Geometry: final body of the model. Coordinates: model frame, mm. Face numbers are marked on the shaded views. Give positions to 0.01 mm unless a question says otherwise; leave off trailing zeros. Loops run counter-clockwise (first coordinate to the right, second up) from the corner with the lowest first, then second, coordinate; pieces in that order, holes last.
```python
from build123d import *

# Parameters (mm, degrees)
SKETCH1_R               = 12.7
BOSS_EXTRUDE1_DEPTH     = 19.05
SHELL1_T                = -3.175
SKETCH4_R               = 1.2446
CUT_EXTRUDE1_DEPTH      = 27.181720723
CUT_EXTRUDE1_DEPTH_BACK = 27.181720723
SKETCH7_R               = 10.8712
SKETCH7_R_2             = 9.525
CUT_EXTRUDE2_DEPTH      = 2.3622


with BuildPart() as part:
    # Sketch1 → Boss-Extrude1 (new body)
    with BuildSketch(Plane.XY):
        Circle(SKETCH1_R)
    extrude(amount=-BOSS_EXTRUDE1_DEPTH)

    # Shell1
    shell1_openings = [part.faces().sort_by_distance(p)[0] for p in [
        (0, 0, -19.05),
    ]]
    offset(amount=SHELL1_T, openings=shell1_openings, kind=Kind.INTERSECTION)

    # Sketch4 → Cut-Extrude1 (cut, two sides)
    with BuildSketch(Plane(origin=(0, 0, 0), x_dir=(0, 0, -1), z_dir=(1, 0, 0))) as cut_extrude1_sk:
        with Locations((13.0175, 0)):
            Circle(SKETCH4_R)
    extrude(amount=CUT_EXTRUDE1_DEPTH, mode=Mode.SUBTRACT)
    extrude(cut_extrude1_sk.sketch, amount=-CUT_EXTRUDE1_DEPTH_BACK, mode=Mode.SUBTRACT)

    # Sketch7 → Cut-Extrude2 (cut)
    with BuildSketch(Plane(origin=(0, 0, -17.78), x_dir=(-1, 0, 0), z_dir=(0, 0, -1))):
        Circle(SKETCH7_R)
        with Locations(Location((0, 0, 0), (0, 0, 180))):
            Circle(SKETCH7_R_2, mode=Mode.SUBTRACT)
    extrude(amount=-CUT_EXTRUDE2_DEPTH, mode=Mode.SUBTRACT)


solid = part.part
```
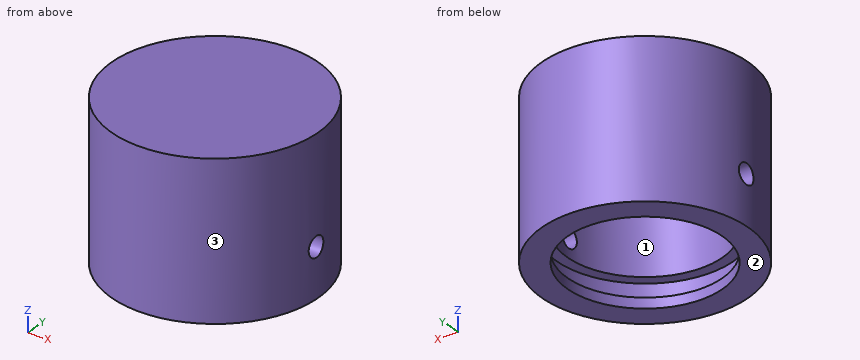
Q1. Mould query, pull axis Y, two halves, no side actions, for the marked faces 1, 2 and 3. Classes: +Y half, -Y half, draft (parallel to the pull), parting line (faces both ways), or undercut.
Q2. Section query C-C, the plane z = -16.25. Return loops of the section in (x, y), and give its area (3 significant figures).
Q3. Section query D-D, the plane z = -13. Return loops of the section in (x, y) (3 decimals), and give its area (3 significant figures).
Q4. Pin query (flat end, axial travel): pin 1 Ø3 at (x, y) = (-2, -5) entering from -Z (3 decimals); pin 2 Ø3 at (x, z) = (-7.5, -9.5) entering from +Y; pin 3 Ø4 at (x, z) = (4.5, -9) entering from +Y. Return the tip coordinate at first contact, or that it passes through.
Q5. Material intervals for probe 1 along Y at (x, z) = (0, -18.4) (3 decimals); probe 2 along Y at (x, z) = (0, -16.55), sorted ascending.
Q6. Section query B-B, the plane x = 0. Return loops of the section in (y, z) (3 decimals), and give its area (3 significant figures).
Q7. Section query A-A, the plane y = 0. Return loops of the section in (x, z) (3 decimals).
Resolved:
1. face 1: undercut
1. face 2: draft
1. face 3: parting line
2. outline: circle Ø25.4 at (0, 0); hole circle Ø21.74 at (0, 0)
2. area: 135 mm2
3. outline: (-12.639, -1.244) arc R12.7 ccw to (12.639, -1.244) - (9.443, -1.244) arc R9.525 cw to (-9.443, -1.244) - close; (-12.639, 1.244) - (-9.443, 1.244) arc R9.525 cw to (9.443, 1.244) - (12.639, 1.244) arc R12.7 ccw to start
3. area: 206 mm2
4. pin 1: stops at z = -3.175
4. pin 2: stops at y = 11.19
4. pin 3: stops at y = 12.45
5. probe 1: y = -12.7 to -9.525, 9.525 to 12.7
5. probe 2: y = -12.7 to -10.87, 10.87 to 12.7
6. outline: (-12.7, -19.05) - (-9.525, -19.05) - (-9.525, -17.78) - (-10.871, -17.78) - (-10.871, -15.418) - (-9.525, -15.418) - (-9.525, -3.175) - (9.525, -3.175) - (9.525, -15.418) - (10.871, -15.418) - (10.871, -17.78) - (9.525, -17.78) - (9.525, -19.05) - (12.7, -19.05) - (12.7, 0) - (-12.7, 0) - close
6. area: 175 mm2
7. outline: (-12.7, -19.05) - (-9.525, -19.05) - (-9.525, -17.78) - (-10.871, -17.78) - (-10.871, -15.418) - (-9.525, -15.418) - (-9.525, -14.262) - (-12.7, -14.262) - close; (-12.7, -11.773) - (-9.525, -11.773) - (-9.525, -3.175) - (9.525, -3.175) - (9.525, -11.773) - (12.7, -11.773) - (12.7, 0) - (-12.7, 0) - close; (9.525, -19.05) - (12.7, -19.05) - (12.7, -14.262) - (9.525, -14.262) - (9.525, -15.418) - (10.871, -15.418) - (10.871, -17.78) - (9.525, -17.78) - close
